Source: CAD feature listing. Evaluate the final solid. Frame: model axes, mm. Face numbers are marked on the shaded views. Round coordinates to 2 decimals unless told otherwise and drop trailing zeros. Order: outer loops, then holes, each group sorted by start corner. A loop starts at its lowest first (then second) coordinate and runs counter-clockwise, first axis right, second up. Notation, with made-up numbers: (50, -37.5) - (84, -37.5) arc R20 cw to (84, -19.5) - close; hole circle Ø11 at (-28, -18.75). An arc over 180 degrees is marked (long way). Put each result on its own line as item: value. Start each with the question number.
1) Line query: probe 1 along Y at (x, z) = (-300, 4.5); probe 2 along Z at (x, y) = (78.5, 50). Output: solid intervals per line, ascending. Write a range as [from, to].
2) Section A-A on x = 384.5. Output: boundary loops of the cut face in (y, z).
3) Contact query for flat-ended pins moving along their axis: P1, Ø10, axis at x = 345.5, z = 58, coming from the +Y side; P2, Ø7.5, axis at x = 15.5, z = 49.5, coming from the +Y side; P3, Ø20, axis at x = -300, y = 50, coming from the +Z side; P4, Ø10, axis at y = 10, z = 47, coming from the +X side. Output: stop coordinate, or through.
4) Section C-C on x = -33. Output: boundary loops of the cut face in (y, z).
5) Mould query, pull axis Y, two halves, no side actions, for the marked faces 1, 2 and 3. Classes: +Y half, -Y half, draft (parallel to the pull), parting line (faces both ways), or undercut.
6) Section B-B on x = -300. Output: boundary loops of the cut face in (y, z).
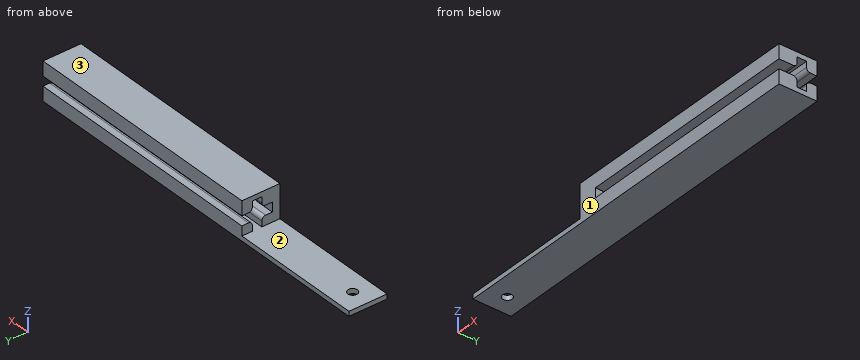
```python
from build123d import *

# Parameters (mm, degrees)
BOSS_EXTRUDE1_DEPTH = 650
SKETCH2_W           = 700
SKETCH2_H           = 25
CUT_EXTRUDE1_DEPTH  = 800
FILLET1_R           = 10
SKETCH3_W           = 12.5
SKETCH3_H           = 100
BOSS_EXTRUDE2_DEPTH = 350
SKETCH4_R           = 12.5
CUT_EXTRUDE2_DEPTH  = 350


with BuildPart() as part:
    # Sketch1 → Boss-Extrude1 (new body)
    with BuildSketch(Plane(origin=(0, 0, 0), x_dir=(0, 0, -1), z_dir=(1, 0, 0))):
        Polygon((-100, 0), (0, 0), (0, 100), (-37.5, 100), (-37.5, 72.5), (-12.5, 72.5), (-12.5, 47.5), (-37.5, 47.5), (-37.5, 20), (-62.5, 20), (-62.5, 47.5), (-87.5, 47.5), (-87.5, 72.5), (-62.5, 72.5), (-62.5, 100), (-100, 100), align=None)
    extrude(amount=BOSS_EXTRUDE1_DEPTH)

    # Sketch2 → Cut-Extrude1 (cut)
    with BuildSketch(Plane.XZ):
        with Locations((400, 50)):
            Rectangle(SKETCH2_W, SKETCH2_H)
    extrude(amount=-CUT_EXTRUDE1_DEPTH, mode=Mode.SUBTRACT)

    # Fillet1
    fillet1_edges = [part.edges().sort_by_distance(p)[0] for p in [
        (325, 72.5, 37.5),
        (325, 72.5, 62.5),
        (325, 47.5, 62.5),
        (325, 47.5, 37.5),
    ]]
    fillet(fillet1_edges, radius=FILLET1_R)

    # Sketch3 → Boss-Extrude2 (add)
    with BuildSketch(Plane.ZY):
        with Locations((6.25, 50)):
            Rectangle(SKETCH3_W, SKETCH3_H)
    extrude(amount=BOSS_EXTRUDE2_DEPTH)

    # Sketch4 → Cut-Extrude2 (cut)
    with BuildSketch(Plane.XY.offset(12.5)):
        with Locations((-300, 50)):
            Circle(SKETCH4_R)
    extrude(amount=-CUT_EXTRUDE2_DEPTH, mode=Mode.SUBTRACT)


solid = part.part
```
Answer sheet:
1. probe 1: [0, 37.5], [62.5, 100]
1. probe 2: [0, 12.5], [87.5, 100]
2. outline: (0, 0) - (100, 0) - (100, 37.5) - (82.5, 37.5) arc R10 ccw to (72.5, 27.5) - (72.5, 12.5) - (47.5, 12.5) - (47.5, 27.5) arc R10 ccw to (37.5, 37.5) - (0, 37.5) - close; (0, 62.5) - (37.5, 62.5) arc R10 ccw to (47.5, 72.5) - (47.5, 87.5) - (72.5, 87.5) - (72.5, 72.5) arc R10 ccw to (82.5, 62.5) - (100, 62.5) - (100, 100) - (0, 100) - close
3. P1: y = 100
3. P2: y = 20
3. P3: through
3. P4: x = 50
4. outline: (0, 0) - (100, 0) - (100, 12.5) - (0, 12.5) - close
5. face 1: -Y half
5. face 2: undercut
5. face 3: draft
6. outline: (0, 0) - (37.5, 0) - (37.5, 12.5) - (0, 12.5) - close; (62.5, 0) - (100, 0) - (100, 12.5) - (62.5, 12.5) - close
